Geometry: final body of the model. Coordinates: model frame, mm. A direction names the side the tool comes from. Give positions to 0.01 mm unless a question says otherwise; leave off trailing zeros. Loops run counter-clockwise (first coordinate to the right, second up) from the corner with the lowest first, then second, coordinate; pieces in that order, holes last. Notation, with made-up numbers: M 17.5,-37 L 35.5,-37 A18 ccw 35.5,-18 Z; hole C 26,89.5 d6. An arc over 180 degrees is marked long. Put each result on its own line as item: value.
```python
from build123d import *

# Parameters (mm, degrees)
SKETCH_1_R               = 16.3
EXTRUDE_1_DEPTH          = 19.75
SKETCH_2_W               = 46.5
SKETCH_2_H               = 2.5
EXTRUDE_2_DEPTH          = 39.5
SKETCH_3_W               = 54.844436064
SKETCH_3_H               = 25.506740045
CUT_EXTRUDE_1_DEPTH      = 50
EXTRUDE_3_DEPTH          = 5.05
SKETCH_5_R               = 14.25
CUT_EXTRUDE_2_DEPTH      = 29.4
SKETCH_6_R               = 2.5
CUT_EXTRUDE_3_DEPTH      = 50.668048079
CUT_EXTRUDE_6_REACH      = 55.295
SKETCH_9_R               = 7.5
SKETCH_12_R              = 1.15
CUT_EXTRUDE_9_DEPTH      = 41.867774591
SKETCH_13_R              = 2
CUT_EXTRUDE_10_DEPTH     = 1
SKETCH_15_W              = 2.8
SKETCH_15_H              = 12
CUT_EXTRUDE_12_DEPTH     = 1.3
EXTRUDE_5_REACH          = 46.665
EXTRUDE_5_END_RADIUS     = 16.3
SKETCH_16_W              = 4
SKETCH_16_H              = 5
SKETCH_17_W              = 1
SKETCH_17_H              = 2
CUT_EXTRUDE_13_DEPTH     = 2.5
SKETCH_19_R              = 8.51898124
SKETCH_19_R_2            = 6.5
EXTRUDE_6_DEPTH          = 2.25
CUT_EXTRUDE_18_REACH     = 55.295
SKETCH_20_R              = 1.15
PATTERN_CIRCULAR_1_COUNT = 4
CUT_EXTRUDE_8_DEPTH      = 54.084861307
SKETCH_18_W              = 26.346157216
SKETCH_18_H              = 2.75
CUT_EXTRUDE_16_DEPTH     = 12.5
FILLET_1_R               = 2
FILLET_2_R               = 1
SKETCH_21_R              = 2.1
CUT_EXTRUDE_19_DEPTH     = 2.5
CUT_EXTRUDE_START        = -10
SKETCH_22_R              = 7.5
CUT_EXTRUDE_23_DEPTH     = 10
EXTRUDE_START            = -1
SKETCH_23_R              = 7.5
SKETCH_23_R_2            = 6.5
EXTRUDE_7_DEPTH          = 1
MOVE_FACE_3_BY           = 0.5
SKETCH_27_W              = 1
SKETCH_27_H              = 39.5
CUT_EXTRUDE_24_DEPTH     = 41.867774591
CHAMFER_1_SIZE           = 2
CHAMFER_1_SIZE2          = 1


with BuildPart() as part:
    # 草图1 → 凸台-拉伸1 (new, symmetric)
    with BuildSketch(Plane(origin=(0, 0, 0), x_dir=(1, 0, 0), z_dir=(0, 1, 0))):
        with Locations(Location((0, 0, 0), (0, 0, 270))):
            Circle(SKETCH_1_R)
    extrude(amount=EXTRUDE_1_DEPTH, both=True)

    # 草图2 → 凸台-拉伸2 (add, through all)
    with BuildSketch(Plane.XZ.offset(19.75)):
        with Locations((8.6, -8.35)):
            Rectangle(SKETCH_2_W, SKETCH_2_H)
    extrude(amount=-EXTRUDE_2_DEPTH)

    # 草图3 → 切除-拉伸1 (cut)
    with BuildSketch(Plane.XZ.offset(19.75)):
        with Locations((4.427781968, 5.653370022)):
            Rectangle(SKETCH_3_W, SKETCH_3_H)
    extrude(amount=-CUT_EXTRUDE_1_DEPTH, mode=Mode.SUBTRACT)

    # 草图4 → 凸台-拉伸3 (add)
    with BuildSketch(Plane.XZ.offset(19.75)):
        with BuildLine():
            Line((-14.65, -7.146152811), (-7.996542478, 4.549209646))
            ThreePointArc((-7.996542478, 4.549209646), (-0.608425307, 9.179859402), (7.326204954, 5.564775015))
            ThreePointArc((7.326204954, 5.564775015), (15.146356853, -2.073759423), (24.85, -7.107773105))
            Line((24.85, -7.107773105), (-14.65, -7.146152811))
        make_face()
    extrude_3 = extrude(amount=-EXTRUDE_3_DEPTH)

    # 镜向1: 凸台-拉伸3 across plane
    add(extrude_3.mirror(Plane.ZX))

    # 草图5 → 切除-拉伸2 (cut)
    with BuildSketch(Plane(origin=(0, -14.7, 0), x_dir=(1, 0, 0), z_dir=(0, 1, 0))):
        Circle(SKETCH_5_R)
    extrude(amount=CUT_EXTRUDE_2_DEPTH, mode=Mode.SUBTRACT)

    # 草图6 → 切除-拉伸3 (cut, through all)
    with BuildSketch(Plane(origin=(0, -14.7, 0), x_dir=(1, 0, 0), z_dir=(0, 1, 0))):
        with Locations(Location((0, 0, 0), (0, 0, 270))):
            Circle(SKETCH_6_R)
    extrude(amount=-CUT_EXTRUDE_3_DEPTH, mode=Mode.SUBTRACT)

    # 草图9 → 切除-拉伸6 (cut, up to next)
    with BuildSketch(Plane(origin=(0, 19.75, 0), x_dir=(1, 0, 0), z_dir=(0, 1, 0)), mode=Mode.PRIVATE) as cut_extrude_6_sk1:
        with Locations(Location((0, 0, 0), (0, 0, 270))):
            Circle(SKETCH_9_R)
    cut_extrude_6_tool1 = extrude(cut_extrude_6_sk1.sketch, amount=-CUT_EXTRUDE_6_REACH, mode=Mode.PRIVATE) & part.part
    add(cut_extrude_6_tool1.solids().sort_by_distance((0, 19.75, 0))[0], mode=Mode.SUBTRACT)

    # 草图12 → 切除-拉伸9 (cut, through all)
    with BuildSketch(Plane.XY.offset(-7.1)):
        with Locations((27.5, 0)):
            Circle(SKETCH_12_R)
    extrude(amount=-CUT_EXTRUDE_9_DEPTH, mode=Mode.SUBTRACT)

    # 草图13 → 切除-拉伸10 (cut)
    with BuildSketch(Plane.XY.offset(-7.1)):
        with Locations((27.5, 0)):
            Circle(SKETCH_13_R)
    extrude(amount=-CUT_EXTRUDE_10_DEPTH, mode=Mode.SUBTRACT)

    # 草图15 → 切除-拉伸12 (cut)
    with BuildSketch(Plane.XY.offset(-7.1)):
        with Locations((-14.672423113, 0)):
            Rectangle(SKETCH_15_W, SKETCH_15_H)
    extrude(amount=-CUT_EXTRUDE_12_DEPTH, mode=Mode.SUBTRACT)

    # 凸台-拉伸5: up to this cylinder (the profile starts outside it)
    extrude_5_end = Plane(origin=(0, 13.4, 0), z_dir=(0, -1, 0)) * Cylinder(EXTRUDE_5_END_RADIUS, 126.93, mode=Mode.PRIVATE)
    # 草图16 → 凸台-拉伸5 (add, up to the surface)
    with BuildSketch(Plane(origin=(0, 0, -15.1), x_dir=(-1, 0, 0), z_dir=(0, 0, -1)), mode=Mode.PRIVATE) as extrude_5_sk1:
        with Locations((11.65, 13.4)):
            Rectangle(SKETCH_16_W, SKETCH_16_H)
    extrude_5_tool1 = extrude(extrude_5_sk1.sketch, amount=-EXTRUDE_5_REACH, mode=Mode.PRIVATE) - extrude_5_end
    extrude_5 = extrude_5_tool1.solids().sort_by_distance((-11.65, 13.4, -15.1))[0]
    add(extrude_5)

    # 镜向4: 凸台-拉伸5 across plane
    add(extrude_5.mirror(Plane.ZX))

    # 草图17 → 切除-拉伸13 (cut)
    with BuildSketch(Plane(origin=(0, 0, -15.1), x_dir=(-1, 0, 0), z_dir=(0, 0, -1))):
        with Locations((11.65, 13.4)):
            Rectangle(SKETCH_17_W, SKETCH_17_H)
    cut_extrude_13 = extrude(amount=-CUT_EXTRUDE_13_DEPTH, mode=Mode.SUBTRACT)

    # 镜向5: 切除-拉伸13 across plane
    add(cut_extrude_13.mirror(Plane.ZX), mode=Mode.SUBTRACT)

    # 草图19 → 凸台-拉伸6 (add)
    with BuildSketch(Plane(origin=(0, 19.75, 0), x_dir=(1, 0, 0), z_dir=(0, 1, 0))):
        Circle(SKETCH_19_R)
        with Locations(Location((0, 0, 0), (0, 0, 270))):
            Circle(SKETCH_19_R_2, mode=Mode.SUBTRACT)
    extrude(amount=-EXTRUDE_6_DEPTH)

    # 草图20 → 切除-拉伸18 (cut, up to next)
    with BuildSketch(Plane.XZ.offset(19.75), mode=Mode.PRIVATE) as cut_extrude_18_sk1:
        with Locations(Location((0, 6, 0), (0, 0, 270))):
            Circle(SKETCH_20_R)
    cut_extrude_18_tool1 = extrude(cut_extrude_18_sk1.sketch, amount=-CUT_EXTRUDE_18_REACH, mode=Mode.PRIVATE) & part.part
    cut_extrude_18 = cut_extrude_18_tool1.solids().sort_by_distance((0, -19.75, 6))[0]
    add(cut_extrude_18, mode=Mode.SUBTRACT)

    # 阵列(圆周)1: 切除-拉伸18 ×4 about axis
    pattern_circular_1_axis = Axis((0, 0, 0), (0, 1, 0))
    for i in range(1, PATTERN_CIRCULAR_1_COUNT):
        add(cut_extrude_18.rotate(pattern_circular_1_axis, i * 360 / PATTERN_CIRCULAR_1_COUNT), mode=Mode.SUBTRACT)

    # 草图7 → 切除-拉伸8 (cut, through all)
    with BuildSketch(Plane.ZY.offset(14.65)):
        Polygon((-7.1, 19.75), (9.2, 18.323934785), (9.2, 19.75), align=None)
    cut_extrude_8 = extrude(amount=-CUT_EXTRUDE_8_DEPTH, mode=Mode.SUBTRACT)

    # 镜向3: 切除-拉伸8 across plane
    add(cut_extrude_8.mirror(Plane.ZX), mode=Mode.SUBTRACT)

    # 草图18 → 切除-拉伸16 (cut)
    with BuildSketch(Plane(origin=(0, 0, -9.6), x_dir=(-1, 0, 0), z_dir=(0, 0, -1))):
        with Locations((0, 18.375)):
            Rectangle(SKETCH_18_W, SKETCH_18_H)
    cut_extrude_16 = extrude(amount=CUT_EXTRUDE_16_DEPTH, mode=Mode.SUBTRACT)

    # 镜向6: 切除-拉伸16 across plane
    add(cut_extrude_16.mirror(Plane.ZX), mode=Mode.SUBTRACT)

    # 圆角1
    fillet_1_edges = [part.edges().sort_by_distance(p)[0] for p in [
        (12.355262037, 0, -7.1),
    ]]
    fillet(fillet_1_edges, radius=FILLET_1_R)

    # 圆角2
    fillet_2_edges = [part.edges().sort_by_distance(p)[0] for p in [
        (-12.355262037, 0, -7.1),
    ]]
    fillet(fillet_2_edges, radius=FILLET_2_R)

    # 草图21 → 切除-拉伸19 (cut)
    with BuildSketch(Plane.XZ.offset(19.75)):
        with Locations(Location((0, 6, 0), (0, 0, 270))):
            Circle(SKETCH_21_R)
        with Locations(Location((-6, 0, 0), (0, 0, 270))):
            Circle(SKETCH_21_R)
        with Locations(Location((6, 0, 0), (0, 0, 270))):
            Circle(SKETCH_21_R)
        with Locations(Location((0, -6, 0), (0, 0, 270))):
            Circle(SKETCH_21_R)
    extrude(amount=-CUT_EXTRUDE_19_DEPTH, mode=Mode.SUBTRACT)

    # 草图22 → 切除-拉伸23 (cut)
    with BuildSketch(Plane.XZ.offset(-17.5).offset(CUT_EXTRUDE_START)):
        with Locations(Location((0, 0, 0), (0, 0, 90))):
            Circle(SKETCH_22_R)
    extrude(amount=CUT_EXTRUDE_23_DEPTH, mode=Mode.SUBTRACT)

    # 草图23 → 凸台-拉伸7 (add)
    with BuildSketch(Plane.XZ.offset(-14.7).offset(EXTRUDE_START)):
        with Locations(Location((0, 0, 0), (0, 0, 288.796905035))):
            Circle(SKETCH_23_R)
        with Locations(Location((0, 0, 0), (0, 0, 270))):
            Circle(SKETCH_23_R_2, mode=Mode.SUBTRACT)
    extrude(amount=EXTRUDE_7_DEPTH)

    # Move Face 3: a face moved outward by 0.5
    extrude(part.faces().sort_by_distance((5.10183032, 14.7, -8.3875))[0], amount=MOVE_FACE_3_BY, dir=(0, -1, 0))

    # 草图27 → 切除-拉伸24 (cut, through all)
    with BuildSketch(Plane.XY.offset(-7.1)):
        with Locations((31.35, 0)):
            Rectangle(SKETCH_27_W, SKETCH_27_H)
    extrude(amount=-CUT_EXTRUDE_24_DEPTH, mode=Mode.SUBTRACT)

    # 倒角1
    chamfer_1_edges = [part.edges().sort_by_distance(p)[0] for p in [
        (30.85, 19.75, -8.35),
    ]]
    chamfer_1_side = [part.faces().sort_by_distance(p)[0] for p in [
        (8.193237095, 19.75, -8.362550861),
    ]]
    chamfer(chamfer_1_edges, length=CHAMFER_1_SIZE, length2=CHAMFER_1_SIZE2, reference=chamfer_1_side[0])


solid = part.part
```
Item 1: Section B-B on z = -12. Output: boundary loops of the cut face in (x, y).
Output values:
outline: M -13.65,-15.9 L -11.03,-15.9 L -11.03,-17 L 11.03,-17 L 11.03,17 L -11.03,17 L -11.03,15.9 L -13.65,15.9 L -13.65,10.9 L -11.03,10.9 L -11.03,-10.9 L -13.65,-10.9 Z; hole M -7.69,-14.7 L 7.69,-14.7 L 7.69,14.2 L -7.69,14.2 Z
Item 2: Line query: probe 1 along Z at (x, y) = (0, -18.5); probe 2 along Y at (x, z) = (-9.5, -9.75); probe 3 along Z at (x, y) = (21.5, -14.5). Output: solid intervals per line, ascending. Write a range as [from, to].
Output values:
probe 1: [-9.6, -8.1], [-3.9, -2.5], [2.5, 3.9]
probe 2: [-17, -14.7], [14.2, 17]
probe 3: [-9.6, -7.1]
Item 3: Mould query, pull axis X, two halves, no side actions, for faces 1 (the cylindrical face through (28.562, -0.44, -8.84)), 2 (the cylindrical face through (15.013, -17.26, -1.977)), 3 (the flat face through (7, 19.75, -8)), 4 (the flat face through (-13.272, 0, -8)). Classes: pulls with the +X half, pulls with the -X half, needs draft (parallel to the pull), parting line crosses it, or undercut.
Output values:
face 1: undercut
face 2: pulls with the +X half
face 3: needs draft
face 4: pulls with the -X half
Item 4: Section C-C on y = -9.5. Output: boundary loops of the cut face in (x, z).
Output values:
outline: M -14.67,-7.1 A16.3 ccw -14.65,-7.15 L -14.65,-9.6 L -13.17,-9.6 A16.3 ccw 13.17,-9.6 L 30.85,-9.6 L 30.85,-7.1 L 13.46,-7.1 A2 ccw 11.81,-7.98 A14.25 cw -12.07,-7.57 A1 ccw -12.92,-7.1 Z
Item 5: Section A-A on y = 0. Output: boundary loops of the cut face in (x, z), then the cut area to 3 significant figures.
Output values:
outline: M -14.65,-9.6 L -13.17,-9.6 A16.3 ccw 13.17,-9.6 L 26.35,-9.6 L 26.35,-8.1 L 25.5,-8.1 L 25.5,-7.1 L 13.46,-7.1 A2 ccw 11.81,-7.98 A14.25 cw -12.07,-7.57 A1 ccw -12.92,-7.1 L -13.27,-7.1 L -13.27,-8.4 L -14.65,-8.4 Z; M 28.65,-9.6 L 30.85,-9.6 L 30.85,-7.1 L 29.5,-7.1 L 29.5,-8.1 L 28.65,-8.1 Z
area: 102 mm²
Item 6: Set-up query: faces 5 (the flat face through (-11.15, 13, -14)), 6 (the flat face through (0, -17, -12)), 7 (the cylindrical face through (-5.369, -18.296, -2.003)), 8 (the flat face through (-14, 6, -8)), 9 (the flat face through (-12, -15.9, -13)). Return all of +Z, -Z, +X, -X, +Y, -Y with unobstructed straight access to the full face (end or side cutting, diameter ignored); none if empty.
Output values:
face 5: -Z
face 6: -Z, +X, -X, -Y
face 7: -Y
face 8: +Z, -X
face 9: -Z, -X, -Y
Item 7: Section D-D on x = 20. Output: boundary loops of the cut face in (y, z), then the cut area to 3 significant figures.
Output values:
outline: M -19.75,-9.6 L 19.75,-9.6 L 19.75,-7.1 L 19.57,-5.05 L 14.2,-5.05 L 14.2,-7.1 L -14.7,-7.1 L -14.7,-5.05 L -19.57,-5.05 L -19.75,-7.1 Z
area: 120 mm²
Item 8: Pin query (flat end, axial travel): pin 1 Ø10 at (x, y) = (8, 6) entering from -Z; pin 2 Ø1.1 at (x, y) = (-11.5, 13.5) entering from -Z; pin 3 Ø12 at (y, z) = (0, -10) entering from -X; pin 4 Ø5 at (x, z) = (-7.5, -12) entering from +Y. Return the tip coordinate at first contact, or that it passes through.
Output values:
pin 1: z = -16.02
pin 2: z = -15.1
pin 3: x = -14.65
pin 4: y = 19.75
